Model file for the job. Use its own axes, mm. Round coordinates to 2 decimals unless told otherwise and drop trailing zeros. Order: outer loops, then holes, each group sorted by start corner. A loop starts at its lowest first (then second) coordinate and runs counter-clockwise, first axis right, second up. Notation, with made-up numbers: (22.25, 15.25) - (67.25, 15.25) arc R17 ccw to (67.25, 40.25) - close; hole circle Ø10 at (81.5, 72). An arc over 180 degrees is marked (long way). Write item = value, one per line.
```python
from build123d import *

# Parameters (mm, degrees)
SKETCH1_W                                       = 539
SKETCH1_H                                       = 299
BOSS_EXTRUDE1_DEPTH                             = 5
SKETCH2_W                                       = 20
SKETCH2_H                                       = 51
CUT_EXTRUDE1_DEPTH                              = 309.229622197
CSK_FOR_M3_FLAT_HEAD_MACHINE_SCREW1_D           = 3.2
CSK_FOR_M3_FLAT_HEAD_MACHINE_SCREW1_CSINK_D     = 6.3
CSK_FOR_M3_FLAT_HEAD_MACHINE_SCREW1_CSINK_ANGLE = 90
LPATTERN1_COUNT                                 = 7
LPATTERN1_PITCH                                 = 85
LPATTERN1_COUNT_DIR2                            = 4
LPATTERN1_PITCH_DIR2                            = 70
CUT_EXTRUDE2_DEPTH                              = 309.229622197
CUT_EXTRUDE3_DEPTH                              = 309.229622197
CUT_EXTRUDE3_DEPTH_BACK                         = 309.229622197
SKETCH6_W                                       = 70
SKETCH6_H                                       = 20
FILLET1_R                                       = 0.5


with BuildPart() as part:
    # Sketch1 → Boss-Extrude1 (new body)
    with BuildSketch(Plane(origin=(0, 0, 0), x_dir=(1, 0, 0), z_dir=(0, 1, 0))):
        Rectangle(SKETCH1_W, SKETCH1_H)
    extrude(amount=BOSS_EXTRUDE1_DEPTH)

    # Sketch2 → Cut-Extrude1 (cut, through all)
    with BuildSketch(Plane(origin=(0, 5, 0), x_dir=(1, 0, 0), z_dir=(0, 1, 0))):
        with Locations((-259.5, 0)):
            Rectangle(SKETCH2_W, SKETCH2_H)
    cut_extrude1 = extrude(amount=-CUT_EXTRUDE1_DEPTH, mode=Mode.SUBTRACT)

    # Mirror1: Cut-Extrude1 across plane
    add(cut_extrude1.mirror(Plane(origin=(0, 0, 0), x_dir=(0, 0, 1), z_dir=(1, 0, 0))), mode=Mode.SUBTRACT)

    # CSK for M3 Flat Head Machine Screw1 (through all)
    with Locations(Plane(origin=(-255, 5, 105), x_dir=(0, 0, 1), z_dir=(0, 1, 0))):
        with Locations((0, 0)):
            csk_for_m3_flat_head_machine_screw1 = CounterSinkHole(CSK_FOR_M3_FLAT_HEAD_MACHINE_SCREW1_D / 2, CSK_FOR_M3_FLAT_HEAD_MACHINE_SCREW1_CSINK_D / 2, counter_sink_angle=CSK_FOR_M3_FLAT_HEAD_MACHINE_SCREW1_CSINK_ANGLE)

    # LPattern1: CSK for M3 Flat Head Machine Screw1 7 × 4
    with Locations(*[(i * LPATTERN1_PITCH, 0, -j * LPATTERN1_PITCH_DIR2) for i in range(LPATTERN1_COUNT) for j in range(LPATTERN1_COUNT_DIR2) if (i, j) != (0, 0)]):
        add(csk_for_m3_flat_head_machine_screw1, mode=Mode.SUBTRACT)

    # Sketch5 → Cut-Extrude2 (cut, through all)
    with BuildSketch(Plane(origin=(0, 5, 0), x_dir=(1, 0, 0), z_dir=(0, 1, 0))):
        with BuildLine():
            Line((-130, -94.5), (-130, 83.5))
            Line((-130, 83.5), (-130, 84.5))
            ThreePointArc((-130, 84.5), (-128.535533906, 88.035533906), (-125, 89.5))
            Line((-125, 89.5), (-115.5, 89.5))
            ThreePointArc((-115.5, 89.5), (-111.964466094, 88.035533906), (-110.5, 84.5))
            Line((-110.5, 84.5), (-110.5, -93.5))
            Line((-110.5, -93.5), (-110.5, -94.5))
            ThreePointArc((-110.5, -94.5), (-111.964466094, -98.035533906), (-115.5, -99.5))
            Line((-115.5, -99.5), (-125, -99.5))
            ThreePointArc((-125, -99.5), (-128.535533906, -98.035533906), (-130, -94.5))
        make_face()
    extrude(amount=-CUT_EXTRUDE2_DEPTH, mode=Mode.SUBTRACT)

    # Sketch6 → Cut-Extrude3 (cut, two sides: drawn at the far end of the back side and taken through both)
    with BuildSketch(Plane(origin=(0, 5, 0), x_dir=(1, 0, 0), z_dir=(0, 1, 0)).offset(-CUT_EXTRUDE3_DEPTH_BACK)):
        Polygon((199.5, 149.5), (199.5, 129.5), (249.5, 129.5), (249.5, 91.5), (269.5, 91.5), (269.5, 149.5), align=None)
        with Locations((234.5, -139.5)):
            Rectangle(SKETCH6_W, SKETCH6_H)
    extrude(amount=CUT_EXTRUDE3_DEPTH + CUT_EXTRUDE3_DEPTH_BACK, mode=Mode.SUBTRACT)

    # Fillet1
    fillet1_edges = [part.edges().sort_by_distance(p)[0] for p in [
        (-269.5, 2.5, 25.5),
        (-269.5, 2.5, -25.5),
        (-249.5, 2.5, -25.5),
        (-249.5, 2.5, 25.5),
        (199.5, 2.5, -149.5),
        (269.5, 2.5, -91.5),
        (249.5, 2.5, -91.5),
        (249.5, 2.5, -129.5),
        (199.5, 2.5, -129.5),
        (269.5, 2.5, 129.5),
        (199.5, 2.5, 149.5),
        (199.5, 2.5, 129.5),
        (269.5, 2.5, -25.5),
        (269.5, 2.5, 25.5),
        (249.5, 2.5, 25.5),
        (249.5, 2.5, -25.5),
        (-269.5, 2.5, -149.5),
        (-269.5, 2.5, 149.5),
    ]]
    fillet(fillet1_edges, radius=FILLET1_R)


solid = part.part
```
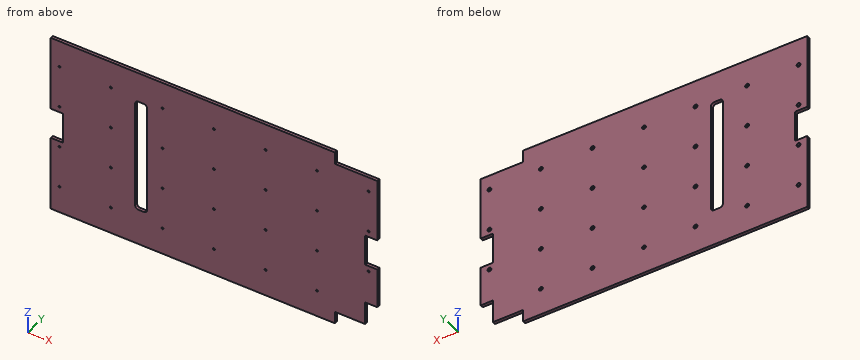
1) Wall check: line 1 along Z through (x, y) = (85, 2.2); line 2 along X through (y, z) = (2.4, -24.5); line 3 along X through (y, z) = (0.95, 71). Give the ranges that are in metal, low to high.
Conclusion:
line_1 = -149.5 to -106.6, -103.4 to -36.6, -33.4 to 33.4, 36.6 to 103.4, 106.6 to 149.5
line_2 = -249.5 to -130, -110.5 to 249.5
line_3 = -269.5 to -130, -110.5 to 269.5
2) Flat gauge pins, fed straight in: pin 1 Ø2.5 at (x, z) = (85, 35) entering from +Y; pin 2 Ø1.5 at (y, z) = (2, -11) entering from +X; pin 3 Ø1.5 at (x, y) = (221, 2) entering from +Z; pin 4 Ø1.5 at (y, z) = (2.5, 144) entering from +X. Where does each tip first touch, or does it go through?
Conclusion:
pin_1 = through
pin_2 = 249.5
pin_3 = 129.5
pin_4 = 199.5
3) Cut at A-A (z = -10.5). Write the cut outline in (x, y), and give its area (3 significant figures).
Conclusion:
outline = (-249.5, 0) - (-130, 0) - (-130, 5) - (-249.5, 5) - close; (-110.5, 0) - (249.5, 0) - (249.5, 5) - (-110.5, 5) - close
area = 2,400 mm^2
4) Cut at B-B (y = 1). Give the number of separate pieces and of enclosed holes in the cut face, and give its area (3 significant figures).
Conclusion:
separate_pieces = 1
enclosed_holes = 28
area = 152,000 mm^2
